For this review, take the finished solid that the model builds, in its own axes (mm). A direction names the side the tool comes from. Coordinates: 2 decimals unless noted, no trailing zeros. Write each loop counter-clockwise with the first axis right and the second up, starting at its lowest first coordinate (ties: lowest second). Pieces come first, ordered by that corner, then holes. Notation, with made-up numbers: (88, 70) -> (109, 70) arc R35 cw to (109, 102) -> close; hole circle Ø6 at (25.5, 20). An arc over 180 degrees is marked (long way). Put each result on its own line as item: value. Start each with the question number.
Item 1: For faces 1 (the cylindrical face through (23.56, 4.68, 19.72)), 2 (the flat face through (-1.3, -16.45, 19.02)), 3 (the flat face through (9, -16.8, 35)), list the 3-axis set-ups (+Z, -Z, +X, -X, +Y, -Y) from which the entire face can be reached by the end or side of a thin tool; tool diameter is ignored.
Item 2: To check wall thickness, follow L1, parallel to Z at x = 7.75, y = -14.1; L2, parallel to Y at x = -15, z = 34.5 (3 decimals); L3, parallel to Z at x = 7, y = -18. State the ranges of each line that lie inside material, in increasing order.
Item 3: The part is to be moulded in two halves that separate along Y. For faces 4 (the cylindrical face through (-13.538, -15.192, 19.72)), 5 (the flat face through (-9, -16.8, 35)), 6 (the flat face through (1.32, -16.45, 19.01)), say which applies: +Y half, -Y half, draft (parallel to the pull), parting line (faces both ways), or undercut.
Item 4: Consider section A-A on y = 15. Give the boundary of the cut face in (x, z) (3 decimals), and give its area (3 significant figures).
Item 5: Consider section B-B on z = 11.5. Give the number of separate pieces and of enclosed holes in the cut face, and give its area (3 significant figures).
Item 6: Consider section D-D on y = -1. Give the boundary of the cut face in (x, z).
Item 7: Insertion check: P1, Ø0.5, axis at x = 15.5, z = 18, coming from the -Y side; P2, Ø0.5, axis at x = 0, z = 38, coming from the +Y side; P3, Ø1.9, axis at x = -8.5, z = 6, coming from the -Y side. Each pin has a flat end and moves straight along its axis. Give the tip position at first contact, or say it passes through.
```python
from build123d import *
from build123d.topology import SkipClean

# Parameters (mm, degrees)
SKETCH1_W             = 60
SKETCH1_H             = 40
BOSS_EXTRUDE1_DEPTH   = 40
SKETCH2_R             = 1.475
CUT_EXTRUDE1_DEPTH    = 54.851648071
LPATTERN1_COUNT       = 6
LPATTERN1_PITCH       = 10
LPATTERN1_COUNT_DIR2  = 4
LPATTERN1_PITCH_DIR2  = 10
SKETCH4_R             = 6.1
CUT_EXTRUDE2_DEPTH    = 65.031242374
SKETCH5_R             = 18.6
CUT_EXTRUDE3_DEPTH    = 33
SKETCH6_R             = 1.5
CUT_EXTRUDE4_DEPTH    = 65.031242374
SKETCH7_R             = 3.1
CUT_EXTRUDE5_DEPTH    = 3
CUT_EXTRUDE6_DEPTH    = 0.2
CIRPATTERN1_COUNT     = 6
CUT_EXTRUDE7_DEPTH    = 33
CUT_EXTRUDE8_DEPTH    = 7
BODY_MOVE_COPY1_ANGLE = 90


with BuildPart() as part:
    # Sketch1 → Boss-Extrude1 (new body)
    with BuildSketch(Plane(origin=(0, 0, 0), x_dir=(1, 0, 0), z_dir=(0, 1, 0))):
        Rectangle(SKETCH1_W, SKETCH1_H)
    extrude(amount=BOSS_EXTRUDE1_DEPTH)

    # Sketch2 → Cut-Extrude1 (cut, through all)
    with BuildSketch(Plane.XZ):
        with Locations(Location((-25, 15, 0), (0, 0, 270))):
            Circle(SKETCH2_R)
    cut_extrude1 = extrude(amount=-CUT_EXTRUDE1_DEPTH, mode=Mode.SUBTRACT)

    # LPattern1: Cut-Extrude1 6 × 4, 14 skipped
    with Locations(*[(i * LPATTERN1_PITCH, 0, -j * LPATTERN1_PITCH_DIR2) for i in range(LPATTERN1_COUNT) for j in range(LPATTERN1_COUNT_DIR2) if (i, j) not in ((0, 0), (1, 1), (1, 2), (1, 3), (2, 0), (2, 1), (2, 2), (2, 3), (3, 0), (3, 1), (3, 2), (3, 3), (4, 1), (4, 2), (4, 3))]):
        add(cut_extrude1, mode=Mode.SUBTRACT)

    # Sketch4 → Cut-Extrude2 (cut, through all)
    with BuildSketch(Plane.XY.offset(20)):
        with Locations((0, 13)):
            Circle(SKETCH4_R)
    extrude(amount=-CUT_EXTRUDE2_DEPTH, mode=Mode.SUBTRACT)

    # Sketch5 → Cut-Extrude3 (cut)
    with BuildSketch(Plane(origin=(0, 0, -20), x_dir=(-1, 0, 0), z_dir=(0, 0, -1))):
        with Locations((0, 20)):
            Circle(SKETCH5_R)
    extrude(amount=-CUT_EXTRUDE3_DEPTH, mode=Mode.SUBTRACT)

    # Sketch6 → Cut-Extrude4 (cut, through all)
    with BuildSketch(Plane.XY.offset(20)):
        with Locations((-15.5, 20)):
            Circle(SKETCH6_R)
    cut_extrude4 = extrude(amount=-CUT_EXTRUDE4_DEPTH, mode=Mode.SUBTRACT)

    # Sketch7 → Cut-Extrude5 (cut)
    with BuildSketch(Plane.XY.offset(20)):
        with Locations((-15.5, 20)):
            Circle(SKETCH7_R)
    cut_extrude5 = extrude(amount=-CUT_EXTRUDE5_DEPTH, mode=Mode.SUBTRACT)

    # Sketch9 → Cut-Extrude6 (cut)
    with SkipClean():  # the faces are left unmerged after this step: merging them gives an invalid solid
        with BuildSketch(Plane.XY.offset(17)):
            with BuildLine():
                Line((-18.212931993, 21.5), (-12.787068007, 21.5))
                ThreePointArc((-12.787068007, 21.5), (-12.4, 20), (-12.787068007, 18.5))
                Line((-12.787068007, 18.5), (-18.212931993, 18.5))
                ThreePointArc((-18.212931993, 18.5), (-18.6, 20), (-18.212931993, 21.5))
            make_face()
        cut_extrude6 = extrude(amount=-CUT_EXTRUDE6_DEPTH, mode=Mode.SUBTRACT)

    # CirPattern1: Cut-Extrude4, Cut-Extrude5, Cut-Extrude6 ×6 about axis
    with SkipClean():  # the faces are left unmerged after this step: merging them gives an invalid solid
        cirpattern1_axis = Axis((0, 20, 0), (0, 0, 1))
        add([cut_extrude4.rotate(cirpattern1_axis, i * 360 / CIRPATTERN1_COUNT) for i in range(1, CIRPATTERN1_COUNT)], mode=Mode.SUBTRACT)
        add([cut_extrude5.rotate(cirpattern1_axis, i * 360 / CIRPATTERN1_COUNT) for i in range(1, CIRPATTERN1_COUNT)], mode=Mode.SUBTRACT)
        add([cut_extrude6.rotate(cirpattern1_axis, i * 360 / CIRPATTERN1_COUNT) for i in range(1, CIRPATTERN1_COUNT)], mode=Mode.SUBTRACT)

    # Sketch10 → Cut-Extrude7 (cut)
    with BuildSketch(Plane(origin=(0, 0, -20), x_dir=(-1, 0, 0), z_dir=(0, 0, -1))):
        Polygon((-6.361574666, 37.478282747), (-2.180690873, 39), (2.180690873, 39), (6.361574666, 37.478282747), align=None)
    extrude(amount=-CUT_EXTRUDE7_DEPTH, mode=Mode.SUBTRACT)

    # Sketch11 → Cut-Extrude8 (cut)
    with BuildSketch(Plane(origin=(0, 0, 13), x_dir=(-1, 0, 0), z_dir=(0, 0, -1))):
        Polygon((-2.086322874, 18.732124987), (-0.526099098, 19.3), (0.526099098, 19.3), (2.086322874, 18.732124987), align=None)
    extrude(amount=-CUT_EXTRUDE8_DEPTH, mode=Mode.SUBTRACT)


with BuildPart() as part_1:
    # Body-Move/Copy1: read off the stored shape, not the designer's step
    # Body-Move/Copy1: moved
    add(part.part.rotate(Axis((0, 0, 0), (1, 0, 0)), BODY_MOVE_COPY1_ANGLE))


solid = part_1.part
```
Return value:
1. face 1: +Z, -Z
1. face 2: +Y, -Y
1. face 3: -Y
2. L1: 0 to 5.08, 8.08 to 31.92, 34.92 to 40
2. L2: -20 to -16.475, -13.525 to 20
2. L3: 0 to 3.57, 9.58 to 30.42, 36.43 to 40
3. face 4: undercut
3. face 5: -Y half
3. face 6: draft
4. outline: (-30, 0) -> (-26.475, 0) -> (-26.475, 40) -> (-30, 40) -> close; (-23.525, 0) -> (23.525, 0) -> (23.525, 40) -> (-23.525, 40) -> close; (26.475, 0) -> (30, 0) -> (30, 40) -> (26.475, 40) -> close; hole (-6.362, 37.478) arc R18.6 ccw (long way) to (6.362, 37.478) -> (2.181, 39) -> (-2.181, 39) -> close
4. area: 1,070 mm^2
5. separate pieces: 2
5. enclosed holes: 10
5. area: 1,160 mm^2
6. outline: (-30, 0) -> (30, 0) -> (30, 40) -> (-30, 40) -> close; hole (-6.36, 37.48) arc R18.6 ccw (long way) to (6.36, 37.48) -> (2.18, 39) -> (-2.18, 39) -> close
7. P1: y = -17
7. P2: y = -13
7. P3: y = -16.8
